Check sheet for the drawn part. Datum: minimum x, y, z corner. Units: mm. Round coordinates to 2 decimals unless told otherwise and drop trailing zeros. Write each loop counter-clockwise with the first axis right and the second up, starting at its lowest first coordinate (ties: lowest second). Pieces come first, ordered by that corner, then holes. Notation, with made-up numbers: (-16.5, 63.25) -> (12.5, 63.25) arc R29 ccw to (12.5, 93.25) -> close; hole circle Ø10 at (50, 27). An arc over 180 degrees is marked (long way). Use CSV: the item, a comma, the result in double quotes.
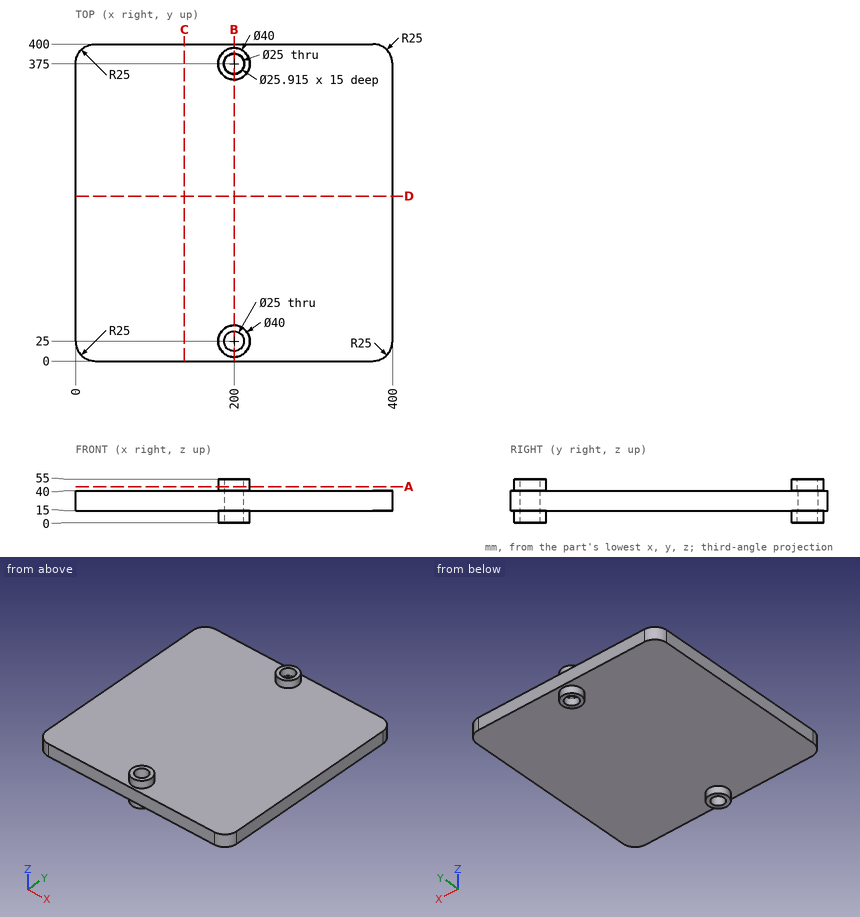
Q1. Section check B-B (x = 200). State how many separate pieces and enclosed holes the cut face has, plus the area to 3 significant figures.
Filled in:
separate pieces,"3"
enclosed holes,"0"
area,"9,620 mm²"
Q2. Material ranges on L1, parallel to Y at x = 200, z = 23; L2, parallel to X at y = 375, z = 5.5; L3, parallel to Y at x = 200, z = 40.5, recorded low to high.
Filled in:
L1,"0 to 12.5, 37.5 to 362.5, 387.5 to 400"
L2,"180 to 187.04, 212.96 to 220"
L3,"5 to 12.5, 37.5 to 45, 355 to 362.04, 387.96 to 395"
Q3. Go/stop test with flat-tipped pins: P1, Ø3, axis at x = 296.5, y = 142.5, coming from the +Z side; P2, Ø12, axis at x = 194, y = 171.5, coming from the -Z side; P3, Ø20.5, axis at x = 200, y = 375, coming from the -Z side. Record where each tip stops, or that it passes through.
Filled in:
P1,"z = 40"
P2,"z = 15"
P3,"through"
Q4. Section check C-C (x = 137.5). Record the cut outline in (y, z), plus the area to 3 significant figures.
Filled in:
outline,"(0, 15) -> (400, 15) -> (400, 40) -> (0, 40) -> close"
area,"10,000 mm²"
Q5. Section check A-A (z = 45.5). Record the cut outline in (x, y) (1 decimal), plus the area to 4 significant figures.
Filled in:
outline,"circle Ø40 at (200, 25); circle Ø40 at (200, 375); hole circle Ø25.9 at (200, 375); hole circle Ø25 at (200, 25)"
area,"1,495 mm²"
